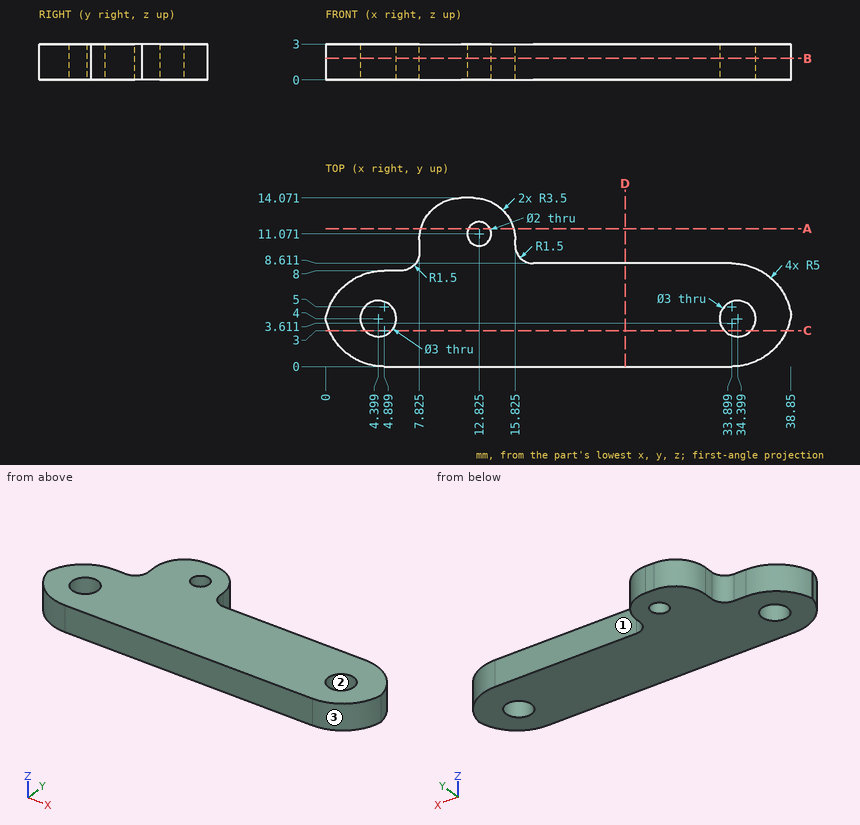
Part print with two shaded views. Sizes in mm from the minimum x, y, z corner. Round coordinates to 2 decimals unless told otherwise and drop trailing zeros. Order: outer loops, then holes, each group sorted by start corner. A loop starts at its lowest first (then second) coordinate and runs counter-clockwise, first axis right, second up. Notation, with made-up numbers: (57, 52.25) -> (65, 52.25) arc R13 cw to (65, 56.25) -> close; hole circle Ø2 at (-22, 5.25). An arc over 180 degrees is marked (long way). One line per question, with ' | ' between items.
Q1. Slice it at A-A (y = 11.5). Write the cut outline in (x, z).
Completed:
outline: (7.95, 0) -> (11.92, 0) -> (11.92, 3) -> (7.95, 3) -> close; (13.73, 0) -> (15.7, 0) -> (15.7, 3) -> (13.73, 3) -> close
Q2. Two-plate mould, pull along Y, no slides. Class the marked faces 1, 2 and 3: released by +Y, released by -Y, zero draft, split by the parting line, or undercut.
Completed:
face 1: released by +Y | face 2: undercut | face 3: released by -Y
Q3. Probe probe 1 along Y at (x, z) = (19, 1.05); probe 2 along Y at (x, z) = (14, 2.3) (1 decimal); probe 3 along X at (y, z) = (6.5, 2.1). List the from-to ranges inside material, lowest first.
Completed:
probe 1: y = 0 to 8.61 | probe 2: y = 0 to 13.6 | probe 3: x = 1.33 to 37.98
Q4. Drop flat-ended pins along their axis: pin 1 (1.2 mm diameter, centred on x = 12.83, y = 11.07, fed in from +Z); pin 2 (0.9 mm diameter, centred on x = 26.5, z = 1.5, fed in from +Y); pin 3 (1.1 mm diameter, centred on x = 5.5, z = 2, fed in from +Y); pin 4 (0.9 mm diameter, centred on y = 10, z = 1.5, fed in from -X) (1 decimal). Give the stop position or say it passes through.
Completed:
pin 1: passes through | pin 2: stops at y = 8.61 | pin 3: stops at y = 8 | pin 4: stops at x = 7.8
Q5. Slice it at B-B (z = 1.8). Give the number of separate pieces and of enclosed holes in the cut face, then the cut area to 3 significant figures.
Completed:
separate pieces: 1 | enclosed holes: 3 | area: 332 mm^2
Q6. Slice it at C-C (y = 3). Write the cut outline in (x, z).
Completed:
outline: (0.32, 0) -> (3.28, 0) -> (3.28, 3) -> (0.32, 3) -> close; (5.52, 0) -> (33.28, 0) -> (33.28, 3) -> (5.52, 3) -> close; (35.52, 0) -> (38.48, 0) -> (38.48, 3) -> (35.52, 3) -> close
Q7. Slice it at D-D (x = 25). Write the cut outline in (y, z).
Completed:
outline: (0, 0) -> (8.61, 0) -> (8.61, 3) -> (0, 3) -> close
